CAD build for the part. Positions are in the model's coordinates, mm. Give positions to 0.01 mm unless a question says otherwise; leave off trailing zeros. Order: outer loops, then holes, each group sorted by start corner. A loop starts at its lowest first (then second) coordinate and runs counter-clockwise, first axis right, second up. Notation, with made-up numbers: (15.5, 22.5) -> (68.5, 22.5) arc R17 ccw to (68.5, 40.5) -> close; hole circle Ø10 at (-18.5, -15.5). An arc over 180 degrees is marked (long way). Use one line per item in the form item = value. Start each with the question number.
1) Cut at A-A, the plane z = 6. Give the cut face in (x, y), and give its area (3 significant figures).
2) Probe line 1 (Z direction, x = -20, y = -13.7); line 2 (Z direction, x = -19.25, y = -11.8); line 3 (Y direction, x = -17, z = 2). List the from-to ranges inside material, lowest first.
3) Cut at B-B, the plane x = -12.25. Give the cut face in (y, z), and give its area (3 significant figures).
4) Cut at C-C, the plane z = 1.25. Give the cut face in (x, y).
5) Mould opens along X. For faces 1 (the face through (-18.86, -12.83, 5.76)), 2 (the face through (-10.33, -13.53, 4.93)), 3 (the face through (-18, -13, 0)) say: pulls with the +X half, pulls with the -X half, needs draft (parallel to the pull), parting line crosses it, or undercut.
6) Drop flat-ended pins along their axis: P1, Ø1.5, axis at x = -14.5, z = 5, coming from the -Y side; P2, Ø3, axis at x = -19.5, z = 2, coming from the +Y side; P3, Ø1, axis at x = -17, z = 5.5, coming from the +Y side. Give the stop position or say it passes through.
from build123d import *

# Parameters (mm, degrees)
SKETCH1_W                 = 15.047570974
SKETCH1_H                 = 10
BOSS_EXTRUDE1_DEPTH       = 3.203817716
DRAFT1_ANGLE              = -0.325763712
F_2_CLEARANCE_HOLE1_D     = 2.5
F_2_CLEARANCE_HOLE1_DEPTH = 4.421800182


with BuildPart() as part:
    # Sketch1 → Boss-Extrude1 (new body)
    with BuildSketch(Plane(origin=(-1.315367261, -15.86205167, 0), x_dir=(0.99657932, -0.082641756, 0), z_dir=(-0.082641756, -0.99657932, 0))):
        with Locations((-16.701480395, 5)):
            Rectangle(SKETCH1_W, SKETCH1_H)
    extrude(amount=-BOSS_EXTRUDE1_DEPTH)

    # Draft1
    draft1_faces = [part.faces().sort_by_distance(p)[0] for p in [
        (-17.694948105, -11.288953517, 5),
    ]]
    draft(draft1_faces, Plane(origin=(-25.192997126, -10.66717467, 0), x_dir=(-1, 0, 0), z_dir=(0, 0, -1)), DRAFT1_ANGLE)

    # #2 Clearance Hole1
    with Locations(Plane(origin=(-1.052360177, -12.690441673, 0), x_dir=(0.99657932, -0.082641756, 0), z_dir=(0.082641756, 0.99657932, 0))):
        with Locations((-18.725265882, -5)):
            Hole(F_2_CLEARANCE_HOLE1_D / 2, depth=F_2_CLEARANCE_HOLE1_DEPTH)


solid = part.part
Result:
q1.outline = (-25.46, -13.86) -> (-20.72, -14.25) -> (-20.46, -11.09) -> (-25.2, -10.7) -> close; (-19.23, -14.38) -> (-10.46, -15.1) -> (-10.2, -11.94) -> (-18.97, -11.22) -> close
q1.area = 42.9 mm²
q2.line_1 = 0 to 3.75, 6.25 to 10
q2.line_2 = 0 to 3.86, 6.14 to 10
q2.line_3 = -14.56 to -11.36
q3.outline = (-14.96, 0) -> (-11.74, 0) -> (-11.8, 10) -> (-14.96, 10) -> close
q3.area = 31.9 mm²
q4.outline = (-25.46, -13.86) -> (-10.46, -15.1) -> (-10.2, -11.92) -> (-25.19, -10.67) -> close
q5.face_1 = undercut
q5.face_2 = pulls with the +X half
q5.face_3 = needs draft
q6.P1 = -14.83
q6.P2 = -11.03
q6.P3 = -11.34
